from build123d import *

# Parameters (mm, degrees)
F1_DEPTH     = 40
F4_DEPTH     = 8
F5_R         = 5
F6_T1_DEPTH  = 78.6190243925
F6_T4_ANGLE  = 141.3037112845
F6_T8_DEPTH  = 68.6190243925
F6_S9_R      = 40
F6_T10_DEPTH = 38
F6_T15_DEPTH = 55.7606094527
F6_S16_R     = 40
F6_T17_DEPTH = 31
F6_T21_DEPTH = 55.7606094527
F6_S22_R     = 40
F6_T23_DEPTH = 31
F6_T25_ANGLE = 141.3037112845
F6_T29_DEPTH = 68.6190243925
F6_S31_R     = 40
F6_T32_DEPTH = 38
F6_T36_DEPTH = 55.7606094527
F6_S37_R     = 40
F6_T38_DEPTH = 31
F6_T42_DEPTH = 55.7606094527
F6_S43_R     = 40
F6_T44_DEPTH = 31
F8_DEPTH     = 40


# Not quite as in the source:
# - a fillet or chamfer that OpenCascade refuses, or shapes differently, is made with other operations: its cross-section is extruded or revolved along the edge and cut away or added


with BuildPart() as f1:
    # F0 (on Front) → F1 (new body)
    with BuildSketch(Plane.XZ):
        Polygon((-25.644130815, 0), (0, 0), (36.0945345553, 0), (31.4589509991, 12.7361611466), (23.9414100328, 10), (0, 75.778483455), align=None)
    extrude(amount=F1_DEPTH)

    # F3 (on face) → F4 (cut, through all)
    with BuildSketch(Plane(origin=(31.8722760891, 0, 11.6005597948), x_dir=(0, 1, 0), z_dir=(0.9396926208, 0, 0.3420201433))):
        with BuildLine():
            Line((-0.635083269, 1.208481717), (-39.364916731, 1.208481717))
            ThreePointArc((-39.364916731, 1.208481717), (-20, -3.791518283), (-0.635083269, 1.208481717))
        make_face()
    extrude(amount=-F4_DEPTH, mode=Mode.SUBTRACT)

    # F5
    f5_edges = [f1.edges().sort_by_distance(p)[0] for p in [
        (0, -20, 75.778483),
    ]]
    fillet(f5_edges, radius=F5_R)

    # F6: chamfer of 5 on 2 edges, made by hand

    # F6_s2 → F6_t1 (cut)
    with BuildSketch(Plane(origin=(18.4446505209, 0, 54.5039975974), x_dir=(0, 1, 0), z_dir=(-0.3205516352, 0, -0.9472310432))):
        Polygon((-35, -24.2909167836), (-40, -19.2909167836), (-40, -24.2909167836), align=None)
        Polygon((-5, -24.2909167836), (0, -19.2909167836), (0, -24.2909167836), align=None)
    extrude(amount=F6_T1_DEPTH, mode=Mode.SUBTRACT)

    # F6_s3 → F6_t4 (revolve, cut)
    with BuildSketch(Plane(origin=(18.4446505209, 0, 54.5039975974), x_dir=(0, 1, 0), z_dir=(-0.3205516352, 0, -0.9472310432))):
        Polygon((0, -19.2909167836), (-5, -24.2909167836), (0, -24.2909167836), align=None)
    revolve(axis=Axis((0.1716952919, 0, 60.6877325166), (0, 1, 0)), revolution_arc=F6_T4_ANGLE, mode=Mode.SUBTRACT)


with BuildPart() as f6_tool6:
    # F6_s7 → F6_t8 (new body)
    with BuildSketch(Plane(origin=(3.9845118306, 0, -10.9473562821), x_dir=(0, 1, 0), z_dir=(-0.3420201433, 0, 0.9396926208))):
        Polygon((0, -20.9177677723), (-5, -25.9177677723), (0, -25.9177677723), align=None)
    extrude(amount=F6_T8_DEPTH)

    # F6_s9 → F6_t10 (intersect, symmetric)
    with BuildSketch(Plane(origin=(21.9888073264, 0, 8.0032713538), x_dir=(0, 1, 0), z_dir=(0.9396926208, 0, 0.3420201433))):
        with Locations((-20, 36.208481717)):
            Circle(F6_S9_R)
    extrude(amount=F6_T10_DEPTH, both=True, mode=Mode.INTERSECT)

    split(bisect_by=Plane(origin=(-0.4133250901, 0, 1.1356013518), x_dir=(0, 1, 0), z_dir=(0.3420201433, 0, -0.9396926208)), keep=Keep.TOP)


with BuildPart() as f1_1:
    add(f1.part)

    # F6_t5: cut F6_tool6
    add(f6_tool6.part, mode=Mode.SUBTRACT)


with BuildPart() as f6_tool13:
    # F6_s14 → F6_t15 (new body)
    with BuildSketch(Plane(origin=(-0.4133250901, 0, 1.1356013518), x_dir=(0, 1, 0), z_dir=(-0.3420201433, 0, 0.9396926208))):
        Polygon((0, -20.9177677723), (-5, -25.9177677723), (0, -25.9177677723), align=None)
    extrude(amount=F6_T15_DEPTH)

    # F6_s16 → F6_t17 (cut, symmetric)
    with BuildSketch(Plane(origin=(21.9888073264, 0, 8.0032713538), x_dir=(0, 1, 0), z_dir=(0.9396926208, 0, 0.3420201433))):
        with Locations((-20, 36.208481717)):
            Circle(F6_S16_R)
    extrude(amount=F6_T17_DEPTH, both=True, mode=Mode.SUBTRACT)


with BuildPart() as f1_2:
    add(f1_1.part)

    # F6_t12: cut F6_tool13
    add(f6_tool13.part, mode=Mode.SUBTRACT)


with BuildPart() as f6_tool19:
    # F6_s20 → F6_t21 (new body)
    with BuildSketch(Plane(origin=(-0.4133250901, 0, 1.1356013518), x_dir=(0, 1, 0), z_dir=(-0.3420201433, 0, 0.9396926208))):
        Polygon((0, -20.9177677723), (-5, -25.9177677723), (0, -25.9177677723), align=None)
    extrude(amount=F6_T21_DEPTH)

    # F6_s22 → F6_t23 (intersect, symmetric)
    with BuildSketch(Plane(origin=(21.9888073264, 0, 8.0032713538), x_dir=(0, 1, 0), z_dir=(0.9396926208, 0, 0.3420201433))):
        with Locations((-20, 36.208481717)):
            Circle(F6_S22_R)
    extrude(amount=F6_T23_DEPTH, both=True, mode=Mode.INTERSECT)


with BuildPart() as f1_3:
    add(f1_2.part)

    # F6_t18: cut F6_tool19
    add(f6_tool19.part, mode=Mode.SUBTRACT)

    # F6_s24 → F6_t25 (revolve, cut)
    with BuildSketch(Plane(origin=(18.4446505209, 0, 54.5039975974), x_dir=(0, 1, 0), z_dir=(-0.3205516352, 0, -0.9472310432))):
        Polygon((-35, -24.2909167836), (-40, -19.2909167836), (-40, -24.2909167836), align=None)
    revolve(axis=Axis((0.1716952919, -40, 60.6877325166), (0, 1, 0)), revolution_arc=F6_T25_ANGLE, mode=Mode.SUBTRACT)


with BuildPart() as f6_tool27:
    # F6_s28 → F6_t29 (new body)
    with BuildSketch(Plane(origin=(3.9845118306, 0, -10.9473562821), x_dir=(0, 1, 0), z_dir=(-0.3420201433, 0, 0.9396926208))):
        Polygon((-40, -20.9177677723), (-35, -25.9177677723), (-40, -25.9177677723), align=None)
    extrude(amount=F6_T29_DEPTH)

    split(bisect_by=Plane(origin=(-0.4133250901, 0, 1.1356013518), x_dir=(0, 1, 0), z_dir=(0.3420201433, 0, -0.9396926208)), keep=Keep.TOP)

    # F6_s31 → F6_t32 (intersect, symmetric)
    with BuildSketch(Plane(origin=(21.9888073264, 0, 8.0032713538), x_dir=(0, 1, 0), z_dir=(0.9396926208, 0, 0.3420201433))):
        with Locations((-20, 36.208481717)):
            Circle(F6_S31_R)
    extrude(amount=F6_T32_DEPTH, both=True, mode=Mode.INTERSECT)


with BuildPart() as f1_4:
    add(f1_3.part)

    # F6_t26: cut F6_tool27
    add(f6_tool27.part, mode=Mode.SUBTRACT)


with BuildPart() as f6_tool34:
    # F6_s35 → F6_t36 (new body)
    with BuildSketch(Plane(origin=(-0.4133250901, 0, 1.1356013518), x_dir=(0, 1, 0), z_dir=(-0.3420201433, 0, 0.9396926208))):
        Polygon((-40, -20.9177677723), (-35, -25.9177677723), (-40, -25.9177677723), align=None)
    extrude(amount=F6_T36_DEPTH)

    # F6_s37 → F6_t38 (cut, symmetric)
    with BuildSketch(Plane(origin=(21.9888073264, 0, 8.0032713538), x_dir=(0, 1, 0), z_dir=(0.9396926208, 0, 0.3420201433))):
        with Locations((-20, 36.208481717)):
            Circle(F6_S37_R)
    extrude(amount=F6_T38_DEPTH, both=True, mode=Mode.SUBTRACT)


with BuildPart() as f1_5:
    add(f1_4.part)

    # F6_t33: cut F6_tool34
    add(f6_tool34.part, mode=Mode.SUBTRACT)


with BuildPart() as f6_tool40:
    # F6_s41 → F6_t42 (new body)
    with BuildSketch(Plane(origin=(-0.4133250901, 0, 1.1356013518), x_dir=(0, 1, 0), z_dir=(-0.3420201433, 0, 0.9396926208))):
        Polygon((-40, -20.9177677723), (-35, -25.9177677723), (-40, -25.9177677723), align=None)
    extrude(amount=F6_T42_DEPTH)

    # F6_s43 → F6_t44 (intersect, symmetric)
    with BuildSketch(Plane(origin=(21.9888073264, 0, 8.0032713538), x_dir=(0, 1, 0), z_dir=(0.9396926208, 0, 0.3420201433))):
        with Locations((-20, 36.208481717)):
            Circle(F6_S43_R)
    extrude(amount=F6_T44_DEPTH, both=True, mode=Mode.INTERSECT)


with BuildPart() as f1_6:
    add(f1_5.part)

    # F6_t39: cut F6_tool40
    add(f6_tool40.part, mode=Mode.SUBTRACT)

    # F7 (on face) → F8 (cut, through all)
    with BuildSketch(Plane.XZ.offset(40)):
        Polygon((2.4692938483, 18.390625), (0, 34), (-2.4692938483, 18.390625), (-13.8564064606, 10), (0, 15.3219454766), (13.8564064606, 10), align=None)
    extrude(amount=-F8_DEPTH, mode=Mode.SUBTRACT)


solid = f1_6.part
CAD build for the part. Positions are in the model's coordinates, mm. Coordinates: 2 decimals unless noted, no trailing zeros. Loops run counter-clockwise (first coordinate to the right, second up) from the corner with the lowest first, then second, coordinate; pieces in that order, holes last. Notation, with made-up numbers: (51.5, 47) -> (57.5, 47) arc R20 ccw to (57.5, 60) -> close; hole circle Ø5 at (53, -39.75). An arc over 180 degrees is marked (long way). One line per item, written item: value.
1. Drill centre lines: line 1 (X direction, y = -14.5, z = 27); line 2 (X direction, y = -16, z = 30.5); line 3 (X direction, y = -19.5, z = 55.5). Where is each one in solid material? Low to high. Write a range as [from, to].
Answers:
line 1: x = [-16.51, -1.11], [1.11, 17.75]
line 2: x = [-15.32, -0.55], [0.55, 16.48]
line 3: x = [-6.86, 7.38]
2. Flat gauge pins, fed straight in: P1, Ø10, axis at y = -18.5, z = 42.5, coming from the +X side; P2, Ø5, axis at x = -2.5, y = -14.5, coming from the +Z side; P3, Ø3, axis at x = 19.5, z = 29.5, coming from the +Y side; P4, Ø8, axis at y = -27.5, z = 37, coming from the +X side. Where does each tip first touch, or does it go through?
Answers:
P1: stops at x = 13.93
P2: stops at z = 65.68
P3: passes through
P4: stops at x = 15.57
3. Slice it at B-B on y = -11.5. Write the cut outline in (x, z), and give its area (3 significant figures).
Answers:
outline: (-25.64, 0) -> (36.09, 0) -> (32.86, 8.9) -> (25.34, 6.16) -> (4.87, 62.4) arc R5 ccw to (-4.56, 62.29) -> close; hole (-13.86, 10) -> (0, 15.32) -> (13.86, 10) -> (2.47, 18.39) -> (0, 34) -> (-2.47, 18.39) -> close
area: 1,940 mm^2
4. Slice it at C-C on z = 32. Write the cut outline in (x, y), and give its area (3 significant figures).
Answers:
outline: (-14.82, -35) -> (-9.54, -40) -> (-0.32, -40) -> (-0.32, 0) -> (-9.54, 0) -> (-14.82, -5) -> close; (0.32, -40) -> (10.61, -40) -> (15.93, -35) -> (15.93, -5) -> (10.61, 0) -> (0.32, 0) -> close
area: 1,150 mm^2
5. Slice it at D-D on z = 45.5. Write the cut outline in (x, y), and give its area (3 significant figures).
Answers:
outline: (-10.25, -35) -> (-4.97, -40) -> (5.7, -40) -> (11.02, -35) -> (11.02, -5) -> (5.7, 0) -> (-4.97, 0) -> (-10.25, -5) -> close
area: 798 mm^2
6. Slice it at A-A on x = -9. Write the cut outline in (y, z).
Answers:
outline: (-40, 0) -> (0, 0) -> (0, 11.87) -> (-40, 11.87) -> close; (-40, 13.58) -> (0, 13.58) -> (0, 33.59) -> (-5, 49.18) -> (-35, 49.18) -> (-40, 33.59) -> close
7. Pull direction Z, two halves, no side cores. Call faces 1 (the face through (-8.083, -20.28, 14.254)), 2 (the face through (12.518, -2.465, 33.974)), 3 (the face through (8.24, -20.28, 14.14)), 4 (the face through (7, -40, 17)): pulls with the +Z half, pulls with the -Z half, needs draft (parallel to the pull), parting line crosses it, or undercut.
Answers:
face 1: undercut
face 2: pulls with the +Z half
face 3: undercut
face 4: needs draft
